Can you work these out from the model? Positions are in its coordinate system, mm. Face numbers are marked on the shaded views. Round coordinates to 2 decimals unless told otherwise and drop trailing zeros. Write each loop counter-clockwise with the first axis right and the second up, starting at its lowest first coordinate (ties: lowest second). Pieces come first, ordered by that corner, then holes. Notation, with made-up numbers: M 74.25,74 L 85.25,74 A14 ccw 85.25,100 Z; hole C 69.5,23 d4. An arc over 180 degrees is marked long. Answer in a Markdown table with one row per item. Add a question column.
(1) Suppose I cut it at A-A, the plane y = 0. Write out the boundary of the cut face in (x, z), then the cut area to 3 significant figures.
(2) If I drill on probe 1 along Y at (x, z) = (0, 10.25); probe 2 along X at (y, z) = (-0.1, 9); probe 3 along Y at (x, z) = (0.2, 19.25), over which ranges is the centre line in solid material (lowest first)?
(3) I'm going to push flat-ended pins straight in: pin 1 (1 mm diameter, centred on y = -2, z = 9.5, fed in from +X); pin 2 (1.5 mm diameter, centred on y = -1.5, z = 10, fed in from +X); pin 3 (2 mm diameter, centred on y = 2, z = 3.5, fed in from -X). Where does each tip first touch, or does it pass through?
(4) Suppose I cut it at C-C, the plane x = 0. Write out the boundary of the cut face in (y, z), then the cut area to 3 significant figures.
(5) Suppose I cut it at B-B, the plane z = 17.75. Write out the boundary of the cut face in (x, y).
(6) If we mould it in two halves opening along X, with no side actions, what happens to the marked faces 1, 2 and 3? For each: released by +X, released by -X, zero draft, split by the parting line, or undercut.
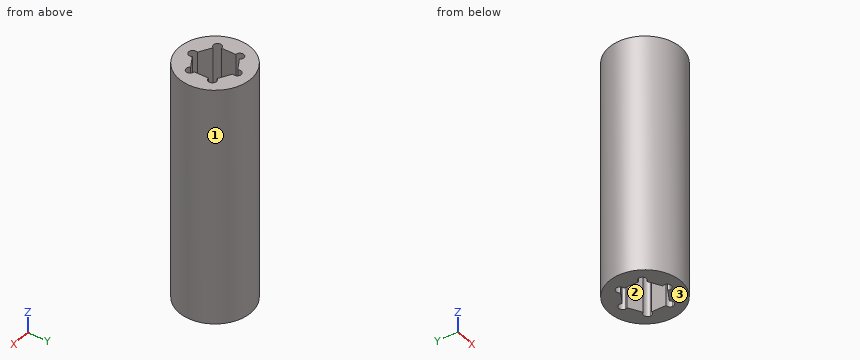
from build123d import *

# Parameters (mm, degrees)
SKETCH1_R           = 3
BOSS_EXTRUDE1_DEPTH = 20


with BuildPart() as part:
    # Sketch1 → Boss-Extrude1 (new body)
    with BuildSketch(Plane.XY):
        Circle(SKETCH1_R)
        with BuildLine():
            Line((-1.309090909, 1.091716873), (-0.290909091, 1.679564419))
            ThreePointArc((-0.290909091, 1.679564419), (-0.086940652, 2.171987791), (0.335912884, 1.847520861))
            ThreePointArc((0.335912884, 1.847520861), (0.32446693, 1.76058021), (0.290909091, 1.679564419))
            Line((0.290909091, 1.679564419), (1.309090909, 1.091716873))
            ThreePointArc((1.309090909, 1.091716873), (1.686940652, 1.248227361), (1.935912884, 0.923760431))
            ThreePointArc((1.935912884, 0.923760431), (1.837526278, 0.686234153), (1.6, 0.587847547))
            Line((1.6, 0.587847547), (1.6, -0.587847547))
            ThreePointArc((1.6, -0.587847547), (1.837526278, -0.686234153), (1.935912884, -0.923760431))
            ThreePointArc((1.935912884, -0.923760431), (1.686940652, -1.248227361), (1.309090909, -1.091716873))
            Line((1.309090909, -1.091716873), (0.290909091, -1.679564419))
            ThreePointArc((0.290909091, -1.679564419), (0.32446693, -1.76058021), (0.335912884, -1.847520861))
            ThreePointArc((0.335912884, -1.847520861), (-0.086940652, -2.171987791), (-0.290909091, -1.679564419))
            Line((-0.290909091, -1.679564419), (-1.309090909, -1.091716873))
            ThreePointArc((-1.309090909, -1.091716873), (-1.890909091, -1.091716873), (-1.6, -0.587847547))
            Line((-1.6, -0.587847547), (-1.6, 0.587847547))
            ThreePointArc((-1.6, 0.587847547), (-1.890909091, 1.091716873), (-1.309090909, 1.091716873))
        make_face(mode=Mode.SUBTRACT)
    extrude(amount=BOSS_EXTRUDE1_DEPTH)


solid = part.part
Calculated:
| question | item | result |
|---|---|---|
| 1 | outline | M -3,0 L -1.6,0 L -1.6,20 L -3,20 Z; M 1.6,0 L 3,0 L 3,20 L 1.6,20 Z |
| 1 | area | 56.0 mm² |
| 2 | probe 1 | -3 to -2.18, 2.18 to 3 |
| 2 | probe 2 | -3 to -1.6, 1.6 to 3 |
| 2 | probe 3 | -2.99 to -2.12, 2.12 to 2.99 |
| 3 | pin 1 | x = 2.6 |
| 3 | pin 2 | x = 2.9 |
| 3 | pin 3 | x = -2.83 |
| 4 | outline | M -3,0 L -2.18,0 L -2.18,20 L -3,20 Z; M 2.18,0 L 3,0 L 3,20 L 2.18,20 Z |
| 4 | area | 32.7 mm² |
| 5 | outline | C 0,0 d6; hole M -1.6,-0.59 A0.34 ccw long -1.31,-1.09 L -0.29,-1.68 A0.34 ccw long 0.29,-1.68 L 1.31,-1.09 A0.34 ccw long 1.6,-0.59 L 1.6,0.59 A0.34 ccw long 1.31,1.09 L 0.29,1.68 A0.34 ccw long -0.29,1.68 L -1.31,1.09 A0.34 ccw long -1.6,0.59 Z |
| 6 | face 1 | split by the parting line |
| 6 | face 2 | undercut |
| 6 | face 3 | zero draft |
